from build123d import *

# Parameters (mm, degrees)
SKETCH1_W           = 48.3
SKETCH1_H           = 58
BOSS_EXTRUDE1_DEPTH = 17
FILLET1_R           = 5
SHELL2_START        = -27.2
SHELL2_DEPTH        = 54.4
SKETCH2_R           = 1.75
CUT_EXTRUDE1_DEPTH  = 17
CHAMFER1_SIZE       = 2.23


# Read off the part's stored shape, not the designer's step: Shell2
with BuildPart() as part:
    # Sketch1 → Boss-Extrude1 (new body)
    with BuildSketch(Plane(origin=(0, 0, 0), x_dir=(1, 0, 0), z_dir=(0, 1, 0))):
        Rectangle(SKETCH1_W, SKETCH1_H)
    extrude(amount=BOSS_EXTRUDE1_DEPTH)

    # Fillet1
    fillet1_edges = [part.edges().sort_by_distance(p)[0] for p in [
        (-24.15, 17, 0),
        (24.15, 17, 0),
    ]]
    fillet(fillet1_edges, radius=FILLET1_R)

    # Shell2 outline → Shell2 (cut)
    with BuildSketch(Plane.XY.offset(SHELL2_START)):
        with BuildLine():
            Line((19.15, 15.2), (19.15, 17))
            Line((19.15, 17), (-19.15, 17))
            Line((-19.15, 17), (-19.15, 15.2))
            ThreePointArc((-19.15, 15.2), (-21.4127417, 14.2627417), (-22.35, 12))
            Line((-22.35, 12), (-22.35, 1.8))
            Line((-22.35, 1.8), (22.35, 1.8))
            Line((22.35, 1.8), (22.35, 12))
            ThreePointArc((22.35, 12), (21.4127417, 14.2627417), (19.15, 15.2))
        make_face()
    extrude(amount=SHELL2_DEPTH, mode=Mode.SUBTRACT)

    # Sketch2 → Cut-Extrude1 (cut)
    with BuildSketch(Plane(origin=(0, 1.8, 0), x_dir=(1, 0, 0), z_dir=(0, 1, 0))):
        with Locations(Location((-15, 0, 0), (0, 0, 270))):
            Circle(SKETCH2_R)
        with Locations(Location((15, 0, 0), (0, 0, 270))):
            Circle(SKETCH2_R)
    extrude(amount=-CUT_EXTRUDE1_DEPTH, mode=Mode.SUBTRACT)

    # Chamfer1
    # the kernel refuses this chamfer: 2.23 mm, written as the material it takes off along each edge
    with BuildSketch(Plane(origin=(-15, 1.8, 0), x_dir=(0, 0, 1), z_dir=(-1, 0, 0))) as chamfer1_piece_1:
        Polygon((1.75, -CHAMFER1_SIZE), (1.75 + CHAMFER1_SIZE, 0), (1.75, 0), align=None)
    revolve(axis=Axis((-15, 1.8, 0), (0, 1, 0)), mode=Mode.SUBTRACT)
    with BuildSketch(Plane(origin=(15, 1.8, 0), x_dir=(0, 0, 1), z_dir=(-1, 0, 0))) as chamfer1_piece_2:
        Polygon((1.75, -CHAMFER1_SIZE), (1.75 + CHAMFER1_SIZE, 0), (1.75, 0), align=None)
    revolve(axis=Axis((15, 1.8, 0), (0, 1, 0)), mode=Mode.SUBTRACT)


solid = part.part
Build history of the part. All positions in model axes, mm. A direction names the side the tool comes from. Round coordinates to 2 decimals unless told otherwise and drop trailing zeros. Write each loop counter-clockwise with the first axis right and the second up, starting at its lowest first coordinate (ties: lowest second). Pieces come first, ordered by that corner, then holes. Notation, with made-up numbers: (-3, 47.5) -> (55, 47.5) arc R22 ccw to (55, 56.5) -> close; hole circle Ø6 at (-38, 86.25). An arc over 180 degrees is marked (long way). Use one line per item in the form item = value.
Q1. Band-saw the part on A-A, the plane z = 0. Write the cut outline in (x, y), then the cut area to 3 significant figures.
Conclusion:
outline = (-24.15, 0) -> (-17.18, 0) -> (-18.98, 1.8) -> (-22.35, 1.8) -> (-22.35, 12) arc R3.2 cw to (-19.15, 15.2) -> (-19.15, 17) arc R5 ccw to (-24.15, 12) -> close; (-12.82, 0) -> (12.82, 0) -> (11.02, 1.8) -> (-11.02, 1.8) -> close; (17.18, 0) -> (24.15, 0) -> (24.15, 12) arc R5 ccw to (19.15, 17) -> (19.15, 15.2) arc R3.2 cw to (22.35, 12) -> (22.35, 1.8) -> (18.98, 1.8) -> close
area = 125 mm²
Q2. Two-plate mould, pull along Z, no slides. Class faces 1 (the flat face through (0, 8, 29)), 2 (the flat face through (0, 10, 27.2)), 3 (the cylindrical face through (22.72, 15.5, -0.41)): released by +Z, released by -Z, zero draft, split by the parting line, or undercut.
Conclusion:
face_1 = released by +Z
face_2 = undercut
face_3 = zero draft
Q3. Band-saw the part on C-C, the plane y = 5.5. Write the cut outline in (x, z), then the cut area to 3 significant figures.
Conclusion:
outline = (-24.15, -29) -> (24.15, -29) -> (24.15, 29) -> (-24.15, 29) -> close; hole (-22.35, -27.2) -> (22.35, -27.2) -> (22.35, 27.2) -> (-22.35, 27.2) -> close
area = 370 mm²
Q4. Tool access for faces 4 (the flat face through (-19.15, 16, 0)), 5 (the flat face through (0, 10, -27.2)), 6 (the cylindrical face through (-22.72, 15.5, -0.41)): list every direction of +Z, -Z, +X, -X, +Y, -Y with a clear straight run to the whole face (end or side of a thin tool).
Conclusion:
face_4 = +Y
face_5 = none
face_6 = +Z, -Z, -X, +Y
Q5. Drill centre lines: L1, parallel to Z at x = -3.5, y = 6; L2, parallel to X at y = 4, z = -16.5; L3, parallel to X at y = 16.5, z = 2. Where is each one in solid material? Low to high.
Conclusion:
L1 = -29 to -27.2, 27.2 to 29
L2 = -24.15 to -22.35, 22.35 to 24.15
L3 = -21.33 to -19.15, 19.15 to 21.33
Q6. Band-saw the part on D-D, the plane z = -7.5. Write the cut outline in (x, y).
Conclusion:
outline = (-24.15, 0) -> (24.15, 0) -> (24.15, 12) arc R5 ccw to (19.15, 17) -> (19.15, 15.2) arc R3.2 cw to (22.35, 12) -> (22.35, 1.8) -> (-22.35, 1.8) -> (-22.35, 12) arc R3.2 cw to (-19.15, 15.2) -> (-19.15, 17) arc R5 ccw to (-24.15, 12) -> close
Q7. Band-saw the part on B-B, the plane x = 15. Write the cut outline in (y, z).
Conclusion:
outline = (0, -29) -> (17, -29) -> (17, -27.2) -> (1.8, -27.2) -> (1.8, -3.98) -> (0, -2.18) -> close; (0, 2.18) -> (1.8, 3.98) -> (1.8, 27.2) -> (17, 27.2) -> (17, 29) -> (0, 29) -> close
Q8. Drop flat-ended pins along their axis: P1, Ø6, axis at x = 4, z = 10.5, coming from the -Y side; P2, Ø1.4, axis at y = 16.5, z = 5, coming from the +X side; P3, Ø2, axis at y = 16.5, z = -13, coming from the -X side. Give the stop position or say it passes through.
Conclusion:
P1 = 0
P2 = 22.4
P3 = -22.72
